Job drawing, mm, ordinate dimensions from the low corner. One solid piece. Give positions to 0.01 mm unless a question says otherwise; leave off trailing zeros. Loops run counter-clockwise (first coordinate to the right, second up) from the corner with the lowest first, then second, coordinate; pieces in that order, holes last. Notation, with made-up numbers: M 18.5,72.25 L 62.5,72.25 A26 ccw 62.5,109.25 Z; hole C -1,68.25 d6. An arc over 180 degrees is marked long. Answer in a Markdown table with one row per item.
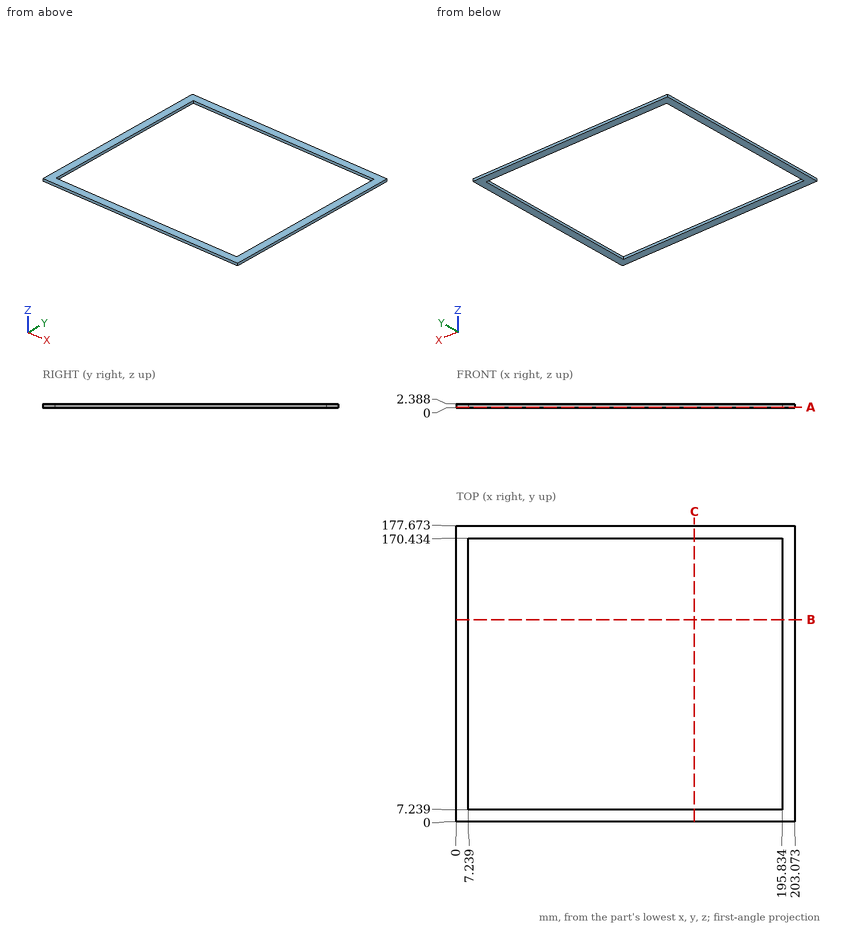
(1) Saw through at C-C (x = 143). Write the cut outline in (y, z).
Recorded:
| item | result |
|---|---|
| outline | M 0,0 L 7.24,0 L 7.24,2.39 L 0,2.39 Z; M 170.43,0 L 177.67,0 L 177.67,2.39 L 170.43,2.39 Z |
(2) Saw through at B-B (y = 121.5). Write the cut outline in (x, z).
Recorded:
| item | result |
|---|---|
| outline | M 0,0 L 7.24,0 L 7.24,2.39 L 0,2.39 Z; M 195.83,0 L 203.07,0 L 203.07,2.39 L 195.83,2.39 Z |
(3) Drill centre lines: line 1 along X through (y, z) = (113, 0.7); line 2 along Y through (x, z) = (40.5, 0.55). Where is each one in solid material? Low to high.
Recorded:
| item | result |
|---|---|
| line 1 | x = 0 to 7.24, 195.83 to 203.07 |
| line 2 | y = 0 to 7.24, 170.43 to 177.67 |
(4) Saw through at A-A (z = 0.5). Write the cut outline in (x, y), plus the area to 3 significant figures.
Recorded:
| item | result |
|---|---|
| outline | M 0,0 L 203.07,0 L 203.07,177.67 L 0,177.67 Z; hole M 7.24,7.24 L 195.83,7.24 L 195.83,170.43 L 7.24,170.43 Z |
| area | 5,300 mm^2 |
